Check sheet for the modelled part. Datum: model origin and axes. Units: mm. Face numbers are marked on the shaded views. A direction names the side the tool comes from. Coordinates: 2 decimals unless noted, no trailing zeros. Write each loop counter-clockwise with the first axis right and the second up, starting at its lowest first coordinate (ties: lowest second). Pieces come first, ordered by that corner, then holes. Notation, with made-up numbers: (68, 85.5) -> (92, 85.5) arc R19 cw to (92, 113.5) -> close; hole circle Ø2 at (32, 32). An arc over 180 degrees is marked (long way). Put each result on its own line as item: value.
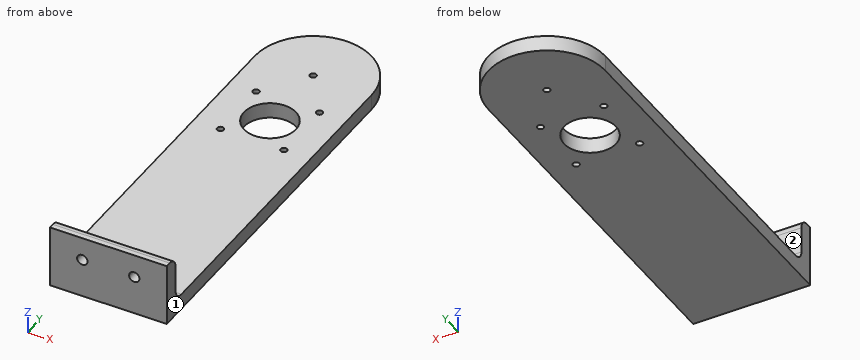
```python
from build123d import *

# Parameters (mm, degrees)
BOSS_EXTRUDE1_DEPTH = 7.62
BOSS_EXTRUDE2_DEPTH = 57.15
FILLET1_R           = 5.08
SKETCH3_R           = 2.54
CUT_EXTRUDE1_DEPTH  = 204.09877166
SKETCH4_R           = 1.5875
CUT_EXTRUDE2_DEPTH  = 183.642823634
SKETCH5_R           = 12.7
CUT_EXTRUDE3_DEPTH  = 183.642823634
SKETCH7_R           = 1.5875
CUT_EXTRUDE4_DEPTH  = 183.642823634


with BuildPart() as part:
    # Sketch1 → Boss-Extrude1 (new body)
    with BuildSketch(Plane.XY):
        with BuildLine():
            Line((-28.575, 0), (-28.575, -177.8))
            Line((-28.575, -177.8), (28.575, -177.8))
            Line((28.575, -177.8), (28.575, 0))
            ThreePointArc((28.575, 0), (0, 28.575), (-28.575, 0))
        make_face()
    extrude(amount=BOSS_EXTRUDE1_DEPTH)

    # Sketch2 → Boss-Extrude2 (add, through all)
    with BuildSketch(Plane.ZY.offset(28.575)):
        with BuildLine():
            Line((0, -177.8), (30.48, -177.8))
            Line((30.48, -177.8), (30.48, -175.26))
            ThreePointArc((30.48, -175.26), (28.992102448, -171.667897552), (25.4, -170.18))
            Line((25.4, -170.18), (0, -170.18))
            Line((0, -170.18), (0, -177.8))
        make_face()
    extrude(amount=-BOSS_EXTRUDE2_DEPTH)

    # Fillet1
    fillet1_edges = [part.edges().sort_by_distance(p)[0] for p in [
        (0, -170.18, 7.62),
    ]]
    fillet(fillet1_edges, radius=FILLET1_R)

    # Sketch3 → Cut-Extrude1 (cut, through all)
    with BuildSketch(Plane(origin=(0, -170.18, 0), x_dir=(1, 0, 0), z_dir=(0, 1, 0))):
        with Locations(Location((12.7, -19.05, 0), (0, 0, 180))):
            Circle(SKETCH3_R)
        with Locations(Location((-12.7, -19.05, 0), (0, 0, 180))):
            Circle(SKETCH3_R)
    extrude(amount=-CUT_EXTRUDE1_DEPTH, mode=Mode.SUBTRACT)

    # Sketch4 → Cut-Extrude2 (cut, through all)
    with BuildSketch(Plane(origin=(0, 0, 0), x_dir=(-1, 0, 0), z_dir=(0, 0, -1))):
        Circle(SKETCH4_R)
    extrude(amount=-CUT_EXTRUDE2_DEPTH, mode=Mode.SUBTRACT)

    # Sketch5 → Cut-Extrude3 (cut, through all)
    with BuildSketch(Plane(origin=(0, 0, 0), x_dir=(-1, 0, 0), z_dir=(0, 0, -1))):
        with Locations((0, -37.465)):
            Circle(SKETCH5_R)
    extrude(amount=-CUT_EXTRUDE3_DEPTH, mode=Mode.SUBTRACT)

    # Sketch7 → Cut-Extrude4 (cut, through all)
    with BuildSketch(Plane(origin=(0, 0, 0), x_dir=(-1, 0, 0), z_dir=(0, 0, -1))):
        with Locations((-15.494, -21.971)):
            Circle(SKETCH7_R)
        with Locations((15.494, -21.971)):
            Circle(SKETCH7_R)
        with Locations((15.494, -52.959)):
            Circle(SKETCH7_R)
        with Locations((-15.494, -52.959)):
            Circle(SKETCH7_R)
    extrude(amount=-CUT_EXTRUDE4_DEPTH, mode=Mode.SUBTRACT)


solid = part.part
```
Q1. Material ranges on line 1 along Y through (x, z) = (0, 3) (1 decimal); line 2 along X through (y, z) = (-172, 19) (1 decimal); line 3 along Z through (x, y) = (-12.7, -175.75), recorded low to high.
Recorded:
line 1: y = -177.8 to -50.2, -24.8 to -1.6, 1.6 to 28.6
line 2: x = -28.6 to -15.2, -10.2 to 10.2, 15.2 to 28.6
line 3: z = 0 to 16.51, 21.59 to 30.48
Q2. Cross-section at D-D (x = -22). Record the cut outline in (y, z), plus the area to 3 significant figures.
Recorded:
outline: (-177.8, 0) -> (18.24, 0) -> (18.24, 7.62) -> (-165.1, 7.62) arc R5.08 cw to (-170.18, 12.7) -> (-170.18, 25.4) arc R5.08 ccw to (-175.26, 30.48) -> (-177.8, 30.48) -> close
area: 1,670 mm2
Q3. Cross-section at A-A (z = 19.05). Record the cut outline in (x, y) (3 decimals), plus the area to 3 significant figures.
Recorded:
outline: (-28.575, -177.8) -> (-15.24, -177.8) -> (-15.24, -170.18) -> (-28.575, -170.18) -> close; (-10.16, -177.8) -> (10.16, -177.8) -> (10.16, -170.18) -> (-10.16, -170.18) -> close; (15.24, -177.8) -> (28.575, -177.8) -> (28.575, -170.18) -> (15.24, -170.18) -> close
area: 358 mm2
Q4. Cross-section at C-C (y = -44). Record the cut outline in (x, z) (3 decimals).
Recorded:
outline: (-28.575, 0) -> (-10.89, 0) -> (-10.89, 7.62) -> (-28.575, 7.62) -> close; (10.89, 0) -> (28.575, 0) -> (28.575, 7.62) -> (10.89, 7.62) -> close
Q5. Cross-section at B-B (x = -4). Record the cut outline in (y, z).
Recorded:
outline: (-177.8, 0) -> (-49.52, 0) -> (-49.52, 7.62) -> (-165.1, 7.62) arc R5.08 cw to (-170.18, 12.7) -> (-170.18, 25.4) arc R5.08 ccw to (-175.26, 30.48) -> (-177.8, 30.48) -> close; (-25.41, 0) -> (28.29, 0) -> (28.29, 7.62) -> (-25.41, 7.62) -> close
Q6. Depth check by flat-ended pin: P1, Ø14, axis at x = -1, z = 20, coming from the +Y side; P2, Ø8, axis at x = 18.5, y = -135, coming from the +Z side; P3, Ø5, axis at x = -7, z = 9.5, coming from the +Y side. Enter the tip coordinate at first touch or a pass-through.
Recorded:
P1: stops at y = -170.18
P2: stops at z = 7.62
P3: stops at y = 28.07
Q7. Tool access check on the marked faces 1 and 2. Record the directions out of +Z, -Z, +X, -X, +Y, -Y that give a thin tool (end or side, any length) a straight path to the whole face; none if there is none.
Recorded:
face 1: +Z, -Z, +X, +Y, -Y
face 2: +Z, +X, -X, +Y
